Source: CAD feature listing. Evaluate the final solid. Frame: model axes, mm. A direction names the side the tool comes from. Give positions to 0.01 mm unless a question says otherwise; leave off trailing zeros. Write each loop counter-clockwise with the first axis right and the second up, starting at its lowest first coordinate (ties: lowest second). Pieces come first, ordered by that corner, then holes. Notation, with made-up numbers: (15.25, 78.5) -> (47.25, 78.5) arc R22 ccw to (47.25, 97.5) -> close; hole circle Ø9 at (-34, 6.25). An arc over 180 degrees is marked (long way). Write item = value, one per line.
Autodesk Inventor part; units mm, degrees
ref_plane "YZ Plane" through (0, 0, 0) normal (1, 0, 0) x (0, 1, 0)
ref_plane "XZ Plane" through (0, 0, 0) normal (0, 1, 0) x (-1, 0, 0)
ref_plane "XY Plane" through (0, 0, 0) normal (0, 0, 1) x (1, 0, 0)
sketch "Sketch1" plane through (0, 0, 0) normal (0, 1, 0) x (-1, 0, 0)
  line L0 (0, 0) -> (60, 0)
  line L1 (60, 0) -> (60, 60)
  line L2 (60, 60) -> (0, 60)
  line L3 (0, 60) -> (0, 0)
  dimension "d0" = 60
  dimension "d1" = 60
extrude "Extrusion1" add sketch "Sketch1" along normal blind 2
sketch "Sketch2" plane through (0, 2, 0) normal (0, 1, 0) x (1, 0, 0)
  line L0 (-60, 0) -> (-60, -60)
  line L1 (-60, -60) -> (0, -60)
  line L2 (0, -60) -> (0, 0)
  line L3 (0, 0) -> (-60, 0)
  line L4 (-58, -2) -> (-58, -58)
  line L5 (-58, -58) -> (-2, -58)
  line L6 (-2, -58) -> (-2, -2)
  line L7 (-2, -2) -> (-58, -2)
  line L8 (-56, -4) -> (-56, -56)
  line L9 (-56, -56) -> (-4, -56)
  line L10 (-4, -56) -> (-4, -4)
  line L11 (-4, -4) -> (-56, -4)
  dimension "d4" = 2
  dimension "d5" = 2
extrude "Extrusion2" add sketch "Sketch2" along normal blind 4 contours L7 L6 L5 L4
sketch "Sketch3" plane through (0, 2, 0) normal (0, 1, 0) x (1, 0, 0)
  line L0 (0, 0) -> (-60, 0) construction
  line L1 (-60, 0) -> (-60, -60) construction
  line L2 (0, 0) -> (-60, -60) construction
  line L3 (-60, -60) -> (0, -60) construction
  line L4 (0, -60) -> (-60, 0) construction
  circle A0 centre (-30, -30) radius 10
  dimension "d8" = 20
hole "Hole1" at (-30, 2, 30) direction (0, -1, 0) diameter 20 depth 8 tip angle 118
sketch "Sketch4" plane through (0, 0, 0) normal (0, -1, 0) x (1, 0, 0)
  circle A0 centre (-30, 30) radius 10
  line L0 (-60, 0) -> (-60, 60)
  line L1 (0, 0) -> (-60, 0)
  line L2 (0, 60) -> (0, 0)
  line L3 (-60, 60) -> (0, 60)
  line L4 (0, 0) -> (-50, 0)
  line L5 (-50, 0) -> (-50, 8)
  line L6 (-50, 8) -> (0, 8)
  line L7 (0, 8) -> (0, 0)
  line L8 (0, 60) -> (-50, 60)
  line L9 (-50, 60) -> (-50, 52)
  line L10 (-50, 52) -> (0, 52)
  line L11 (0, 52) -> (0, 60)
  line L12 (0, 8) -> (-5, 8)
  line L13 (-5, 8) -> (-5, 52)
  line L14 (-5, 52) -> (0, 52)
  line L15 (0, 52) -> (0, 8)
  dimension "d16" = 50
  dimension "d17" = 8
  dimension "d18" = 50
  dimension "d19" = 8
  dimension "d20" = 5
extrude "Extrusion3" add sketch "Sketch4" along normal blind 10 contours L5 L6 L2 L1 | L3 L2 L10 L9 | L6 L13 L10 L2
sketch "Sketch5" plane through (-5, 0, 52) normal (0, 0, -1) x (-1, 0, 0)
  line L0 (55, 0) -> (45, 0)
  line L1 (45, 0) -> (45, -10)
  line L2 (-5, -10) -> (45, -10)
  line L3 (-5, -10) -> (-5, 2)
  line L4 (55, 2) -> (-5, 2)
  line L5 (55, 0) -> (55, 2)
  line L6 (-5, -10) -> (45, -10) construction
  line L7 (-5, -10) -> (5, -10) construction
  line L8 (5, -10) -> (20, -10) construction
  line L9 (20, -10) -> (20, -25) construction
  circle A0 centre (20, -25) radius 15
  point P0 (-5, 0)
  dimension "d23" = 10
  dimension "d24" = 15
  dimension "d25" = 15
  dimension "d26" = 30
extrude "Extrusion4" add sketch "Sketch5" against normal blind 8 contours A0
sketch "Sketch6" plane through (-50, 0, 8) normal (0, 0, 1) x (1, 0, 0)
  line L0 (0, 0) -> (-10, 0)
  line L1 (-10, 0) -> (-10, 2)
  line L2 (50, 2) -> (-10, 2)
  line L3 (50, -10) -> (50, 2)
  line L4 (0, -10) -> (50, -10)
  line L5 (0, 0) -> (0, -10)
  line L6 (0, -10) -> (50, -10) construction
  line L7 (50, -10) -> (40, -10) construction
  line L8 (40, -10) -> (25, -10) construction
  line L9 (25, -10) -> (25, -25) construction
  circle A0 centre (25, -25) radius 15
  point P0 (50, 0)
  dimension "d29" = 10
  dimension "d30" = 15
  dimension "d31" = 15
  dimension "d32" = 30
extrude "Extrusion5" add sketch "Sketch6" against normal blind 8 contours A0
sketch "Sketch7" plane through (-25, -25, 52) normal (0, 0, -1) x (-1, 0, 0)
  circle A0 centre (0, 0) radius 15
  circle A1 centre (0, 0) radius 13.5
  circle A2 centre (0, 0) radius 11.5
  circle A3 centre (0, 0) radius 15
  circle A4 centre (0, 0) radius 15
  line L0 (0, -15) -> (0, 15)
  line L1 (15, 0) -> (-15, 0)
  line L2 (0, 0) -> (-12.9904, -7.5)
  line L3 (0, 0) -> (15, 0) construction
  line L4 (-12.9904, -7.5) -> (12.9904, 7.5)
  line L5 (0, 0) -> (-7.5, -12.9904)
  line L6 (0, 0) -> (15, 0) construction
  line L7 (-7.5, -12.9904) -> (7.5, 12.9904)
  line L8 (0, 0) -> (7.5, -12.9904)
  line L9 (0, 0) -> (15, 0) construction
  line L10 (7.5, -12.9904) -> (-7.5, 12.9904)
  line L11 (0, 0) -> (12.9904, -7.5)
  line L12 (0, 0) -> (15, 0) construction
  line L13 (12.9904, -7.5) -> (-12.9904, 7.5)
  point P0 (-25, 25)
  point P1 (11.6913, 6.75)
  point P2 (9.9593, 5.75)
  point P3 (11.5, 0)
  point P4 (13.5, 0)
  point P5 (5.75, 9.9593)
  point P6 (6.75, 11.6913)
  point P7 (0, 13.5)
  point P8 (0, 11.5)
  point P9 (-11.6913, 6.75)
  point P10 (-9.9593, 5.75)
  point P11 (-5.75, 9.9593)
  point P12 (-6.75, 11.6913)
  point P13 (-11.6913, -6.75)
  point P14 (-9.9593, -5.75)
  point P15 (-11.5, 0)
  point P16 (-13.5, 0)
  point P17 (-5.75, -9.9593)
  point P18 (-6.75, -11.6913)
  point P19 (0, -13.5)
  point P20 (0, -11.5)
  point P21 (11.6913, -6.75)
  point P22 (9.9593, -5.75)
  point P23 (5.75, -9.9593)
  point P24 (6.75, -11.6913)
  dimension "d35" = 1.5
  dimension "d36" = 2
  dimension "d37" = 30
  dimension "d38" = 150
  dimension "d39" = 120
  dimension "d40" = 60
  dimension "d41" = 30
extrude "Extrusion6" cut sketch "Sketch7" against normal blind 5 contours L1 A2 L4 A1 | A1 L8 A2 L11 | L7 A2 L0 A1 | A1 L5 A2 L0 | A2 L2 A1 L1 | A2 L13 A1 L10
sketch "Sketch8" plane through (-25, -25, 8) normal (0, 0, 1) x (1, 0, 0)
  circle A0 centre (0, 0) radius 15
  circle A1 centre (0, 0) radius 13.5
  circle A2 centre (0, 0) radius 11.5
  circle A3 centre (0, 0) radius 15
  circle A4 centre (0, 0) radius 15
  line L0 (0, -15) -> (0, 15)
  line L1 (15, 0) -> (-15, 0)
  line L2 (0, 0) -> (-12.9904, -7.5)
  line L3 (0, 0) -> (15, 0) construction
  line L4 (-12.9904, -7.5) -> (12.9904, 7.5)
  line L5 (0, 0) -> (-7.5, -12.9904)
  line L6 (0, 0) -> (15, 0) construction
  line L7 (-7.5, -12.9904) -> (7.5, 12.9904)
  line L8 (0, 0) -> (7.5, -12.9904)
  line L9 (0, 0) -> (15, 0) construction
  line L10 (7.5, -12.9904) -> (-7.5, 12.9904)
  line L11 (0, 0) -> (12.9904, -7.5)
  line L12 (0, 0) -> (15, 0) construction
  line L13 (12.9904, -7.5) -> (-12.9904, 7.5)
  point P0 (25, 25)
  point P1 (-25, 25)
  point P2 (11.6913, 6.75)
  point P3 (9.9593, 5.75)
  point P4 (11.5, 0)
  point P5 (13.5, 0)
  point P6 (5.75, 9.9593)
  point P7 (6.75, 11.6913)
  point P8 (0, 13.5)
  point P9 (0, 11.5)
  point P10 (-11.6913, 6.75)
  point P11 (-9.9593, 5.75)
  point P12 (-5.75, 9.9593)
  point P13 (-6.75, 11.6913)
  point P14 (-11.6913, -6.75)
  point P15 (-9.9593, -5.75)
  point P16 (-11.5, 0)
  point P17 (-13.5, 0)
  point P18 (-5.75, -9.9593)
  point P19 (-6.75, -11.6913)
  point P20 (0, -13.5)
  point P21 (0, -11.5)
  point P22 (11.6913, -6.75)
  point P23 (9.9593, -5.75)
  point P24 (5.75, -9.9593)
  point P25 (6.75, -11.6913)
  point P26 (9.9593, -5.75)
  point P27 (11.6913, -6.75)
  point P28 (13.5, 0)
  point P29 (11.5, 0)
  point P30 (6.75, 11.6913)
  point P31 (5.75, 9.9593)
  point P32 (9.9593, 5.75)
  point P33 (11.6913, 6.75)
  point P34 (-6.75, 11.6913)
  point P35 (-5.75, 9.9593)
  point P36 (0, 11.5)
  point P37 (0, 13.5)
  point P38 (-9.9593, 5.75)
  point P39 (-11.6913, 6.75)
  point P40 (-13.5, 0)
  point P41 (-11.5, 0)
  point P42 (-6.75, -11.6913)
  point P43 (-5.75, -9.9593)
  point P44 (-9.9593, -5.75)
  point P45 (-11.6913, -6.75)
  point P46 (6.75, -11.6913)
  point P47 (5.75, -9.9593)
  point P48 (0, -11.5)
  point P49 (0, -13.5)
  dimension "d44" = 1.5
  dimension "d45" = 2
  dimension "d46" = 30
  dimension "d47" = 150
  dimension "d48" = 120
  dimension "d49" = 60
  dimension "d50" = 30
extrude "Extrusion7" cut sketch "Sketch8" against normal blind 5 contours A1 L11 A2 L1 | L4 A2 L7 A1 | A1 L0 A2 L8 | L0 A2 L10 A1 | L1 A1 L13 A2 | A2 L5 A1 L2
sketch "Sketch9" plane through (-25, -25, 52) normal (0, 0, -1) x (-1, 0, 0)
  circle A0 centre (0, 0) radius 15
  circle A1 centre (0, 0) radius 7.5
  point P0 (-25, 25)
  point P1 (0, 15)
  dimension "d53" = 15
hole "Hole2" at (-25, -25, 52) direction (0, 0, 1) diameter 15 depth 8 tip angle 118
sketch "Sketch10" plane through (-25, -25, 8) normal (0, 0, 1) x (1, 0, 0)
  circle A0 centre (0, 0) radius 15
  point P0 (25, 25)
  point P1 (0, 15)
hole "Hole3" at (-25, -25, 8) direction (0, 0, -1) diameter 15 depth 8 tip angle 118
sketch "Sketch11" plane through (-25, -25, 8) normal (0, 0, 1) x (1, 0, 0)
  circle A0 centre (0, 0) radius 7.5
  circle A1 centre (0, 0) radius 15
  circle A2 centre (0, 0) radius 9.5
  point P0 (25, 25)
  point P1 (0, 15)
  dimension "d68" = 2
extrude "Extrusion8" cut sketch "Sketch11" against normal blind 6 contours A2
sketch "Sketch12" plane through (-25, -25, 52) normal (0, 0, -1) x (-1, 0, 0)
  circle A0 centre (0, 0) radius 7.5
  circle A1 centre (0, 0) radius 15
  circle A2 centre (0, 0) radius 9.5
  point P0 (-25, 25)
  point P1 (0, 15)
  dimension "d71" = 2
extrude "Extrusion9" cut sketch "Sketch12" against normal blind 6 contours A2
sketch "Sketch13" plane through (-60, 2, 60) normal (0, 0, 1) x (1, 0, 0)
  point P0 (60, -2)
sketch "Sketch14" plane through (-60, 2, 60) normal (0, 0, 1) x (1, 0, 0)
  line L0 (0, -2) -> (10, -2)
  line L1 (10, -2) -> (10, -12)
  line L2 (35, -12) -> (10, -12)
  line L3 (60, -12) -> (35, -12)
  line L4 (60, -12) -> (60, 0)
  line L5 (0, 0) -> (60, 0)
  line L6 (0, -2) -> (0, 0)
  arc A0 (44.9593, -21.25) -> (40.75, -17.0407) centre (35, -27) ccw
  circle A1 centre (35, -27) radius 15
  line L7 (60, -12) -> (60, 0)
  line L8 (60, -12) -> (35, -12)
  line L9 (35, -42) -> (35, -52)
  line L10 (35, -52) -> (60, -52)
  line L11 (60, -52) -> (60, -12)
  arc A2 (35, -42) -> (35, -12) centre (35, -27) ccw
  point P0 (60, -2)
  dimension "d74" = 25
  dimension "d75" = 40
extrude "Extrusion10" add sketch "Sketch14" against normal blind 8 contours L3 L11 L10 L9 A1
sketch "Sketch15" plane through (0, 2, 0) normal (0, 0, -1) x (-1, 0, 0)
  line L0 (50, -2) -> (60, -2)
  line L1 (60, -2) -> (60, 0)
  line L2 (0, 0) -> (60, 0)
  line L3 (0, -12) -> (0, 0)
  line L4 (25, -12) -> (0, -12)
  line L5 (50, -12) -> (25, -12)
  line L6 (50, -2) -> (50, -12)
  circle A0 centre (25, -27) radius 15
  line L7 (0, -52) -> (25, -52)
  line L8 (25, -12) -> (0, -12)
  line L9 (0, -12) -> (0, -52)
  line L10 (0, -52) -> (25, -52)
  circle A1 centre (25, -27) radius 7.5
  arc A2 (25, -12) -> (25, -42) centre (25, -27) ccw
  line L11 (25, -52) -> (25, -42)
  point P0 (0, -2)
extrude "Extrusion11" add sketch "Sketch15" against normal blind 8 contours A0 L11 L7 L9 L4
sketch "Sketch16" plane through (0, -10, 0) normal (0, -1, 0) x (1, 0, 0)
  line L0 (-4, 56) -> (-4, 4)
  line L1 (0, 8) -> (0, 52)
  line L2 (-5, 52) -> (-5, 8)
  line L3 (-25, 8) -> (0, 8)
  line L4 (0, 52) -> (-25, 52)
  line L5 (-5, 8) -> (-5, 52)
  line L6 (0, 8) -> (-5, 8)
  line L7 (-5, 8) -> (-5, 52)
  line L8 (-5, 52) -> (0, 52)
  line L9 (0, 52) -> (0, 8)
  point P0 (0, 0)
extrude "Extrusion12" add sketch "Sketch16" along normal blind 40
sketch "Sketch17" plane through (0, 0, 0) normal (0, -1, 0) x (1, 0, 0)
  line L0 (-50, 52) -> (-50, 60)
  line L1 (-60, 60) -> (-50, 60)
  line L2 (-60, 0) -> (-60, 60)
  line L3 (-50, 0) -> (-60, 0)
  line L4 (-50, 0) -> (-50, 8)
  line L5 (-50, 8) -> (-5, 8)
  line L6 (-5, 8) -> (-5, 52)
  line L7 (-5, 52) -> (-50, 52)
  circle A0 centre (-30, 30) radius 10
  line L8 (-50, 60) -> (-50, 52)
  line L9 (-50, 60) -> (-55, 60)
  line L10 (-55, 60) -> (-55, 0)
  line L11 (-55, 0) -> (-50, 0)
  line L12 (-50, 0) -> (-50, 60)
  point P0 (0, 0)
  dimension "d82" = 5
  dimension "d83" = 60
extrude "Extrusion13" add sketch "Sketch17" along normal blind 20 contours L12 L4 L3 L10 L1 L0
sketch "Sketch18" plane through (0, 2, 0) normal (0, 0, -1) x (-1, 0, 0)
  circle A0 centre (25, -27) radius 7.5
  line L0 (55, -2) -> (60, -2)
  line L1 (60, -2) -> (60, 0)
  line L2 (0, 0) -> (60, 0)
  line L3 (0, -52) -> (0, 0)
  line L4 (0, -52) -> (25, -52)
  line L5 (25, -52) -> (25, -42)
  arc A1 (25, -42) -> (25, -12) centre (25, -27) ccw
  line L6 (50, -12) -> (25, -12)
  line L7 (50, -12) -> (50, -22)
  line L8 (55, -22) -> (50, -22)
  line L9 (55, -2) -> (55, -22)
  line L10 (50, -12) -> (50, -22)
  line L11 (50, -12) -> (25, -12)
  line L12 (50, -22) -> (50, -12)
  arc A2 (39.1421, -22) -> (25, -12) centre (25, -27) ccw
  line L13 (39.1421, -22) -> (50, -22)
  point P0 (0, -2)
extrude "Extrusion14" add sketch "Sketch18" against normal blind 8 contours L13 A1 L6 L7
sketch "Sketch19" plane through (-60, 2, 60) normal (0, 0, 1) x (1, 0, 0)
  circle A0 centre (35, -27) radius 7.5
  arc A1 (35, -12) -> (35, -42) centre (35, -27) ccw
  line L0 (35, -42) -> (35, -52)
  line L1 (35, -52) -> (60, -52)
  line L2 (60, -52) -> (60, 0)
  line L3 (0, 0) -> (60, 0)
  line L4 (0, -2) -> (0, 0)
  line L5 (0, -2) -> (5, -2)
  line L6 (5, -2) -> (5, -22)
  line L7 (10, -22) -> (5, -22)
  line L8 (10, -12) -> (10, -22)
  line L9 (35, -12) -> (10, -12)
  line L10 (35, -22) -> (35, -19.5)
  line L11 (35, -12) -> (10, -12)
  line L12 (10, -12) -> (10, -22)
  arc A2 (35, -12) -> (20.8579, -22) centre (35, -27) ccw
  line L13 (10, -22) -> (20.8579, -22)
  point P0 (60, -2)
extrude "Extrusion15" add sketch "Sketch19" against normal blind 8 contours A1 L13 L8 L9
fillet "Fillet1" radius 5 14 edges at (0, -24, 0) (-55, -10, 0) (-55, -10, 60) (0, -24, 60) (-2, 4, 58) (-2, 4, 2) (-60, 1, 0) (-58, 4, 2) (-60, 1, 60) (-58, 4, 58) (-56, 4, 56) (-56, 4, 4) (-4, 4, 56) (-4, 4, 4)
properties part number "Pieza 2.3 final"
1) Cut plane B-B (z = 16). Return the cut outline in (x, y).
Computed:
outline = (-60, 0) -> (-55, 0) -> (-55, -20) -> (-50, -20) -> (-50, 0) -> (-5, 0) -> (-5, -50) -> (0, -50) -> (0, 2) -> (-2, 2) -> (-2, 6) -> (-4, 6) -> (-4, 2) -> (-56, 2) -> (-56, 6) -> (-58, 6) -> (-58, 2) -> (-60, 2) -> close
2) Cut plane D-D (y = 3). Return the cut outline in (x, z), then the cut area to 3 significant figures.
Computed:
outline = (-58, 7) arc R5 ccw to (-53, 2) -> (-7, 2) arc R5 ccw to (-2, 7) -> (-2, 53) arc R5 ccw to (-7, 58) -> (-53, 58) arc R5 ccw to (-58, 53) -> close; hole (-56, 9) arc R5 ccw to (-51, 4) -> (-9, 4) arc R5 ccw to (-4, 9) -> (-4, 51) arc R5 ccw to (-9, 56) -> (-51, 56) arc R5 ccw to (-56, 51) -> close
area = 432 mm²
3) Cut plane A-A (y = -10.5). Return the cut outline in (x, z).
Computed:
outline = (-55, 5) arc R5 ccw to (-50, 0) -> (-5, 0) arc R5 ccw to (0, 5) -> (0, 55) arc R5 ccw to (-5, 60) -> (-50, 60) arc R5 ccw to (-55, 55) -> close; hole (-50, 8) -> (-5, 8) -> (-5, 52) -> (-50, 52) -> close
4) Cut plane C-C (x = -45). Return the cut outline in (y, z), then the cut area to 3 significant figures.
Computed:
outline = (-20, 0) -> (2, 0) -> (2, 2) -> (6, 2) -> (6, 4) -> (2, 4) -> (2, 56) -> (6, 56) -> (6, 58) -> (2, 58) -> (2, 60) -> (-20, 60) -> (-20, 52) -> (0, 52) -> (0, 8) -> (-20, 8) -> close
area = 456 mm²
5) Material intervals for L1, parallel to Z at x = -18.5, y = -34; L2, parallel to Y at x = -26.5, z = 5; L3, parallel to X at y = -9, z = 47.5, sorted ascending.
Computed:
L1 = 0 to 8, 52 to 60
L2 = -39.92 to -34.38, -15.62 to -13.6, -11.58 to 2
L3 = -55 to -50, -5 to 0
6) Contact query for flat-ended pins moving along their axis: pin 1 (4 mm diameter, centred on x = -38, z = 50, fed in from +Y); pin 2 (2 mm diameter, centred on y = 4.5, z = 38.5, fed in from +X); pin 3 (1.5 mm diameter, centred on y = -4.5, z = 11.5, fed in from -X); pin 4 (13.5 mm diameter, centred on x = -25, y = -25, fed in from +Z). Output: stop coordinate, or through.
Computed:
pin_1 = 2
pin_2 = -2
pin_3 = -55
pin_4 = through
7) Draft query along Z for faces 1 (the cylindrical face through (-2, -24, 1)), 2 (the cylindrical face through (-11.973, -28.542, 5.535)), 3 (the flat face through (-17, 0, 30)), 4 (the cylindrical face through (-1, -24, 58)). Return one class per face: pulls with the +Z half, pulls with the -Z half, needs draft (parallel to the pull), parting line crosses it, or undercut.
Computed:
face_1 = pulls with the -Z half
face_2 = undercut
face_3 = undercut
face_4 = pulls with the +Z half
8) Access query for faces 5 (the flat face through (0, -24, 30)), 6 (the cylindrical face through (-53, -10, 59)), 7 (the cylindrical face through (-28.45, -11.95, 5.54)). Directions: +Z, -Z, +X, -X, +Y, -Y. A direction counts if a zero-diameter tool reaches every point of the face in a straight line with its end or side. Return the directions, or none.
Computed:
face_5 = +Z, -Z, +X, +Y, -Y
face_6 = +Z, -X, -Y
face_7 = none
